```python
from build123d import *

# Parameters (mm, degrees)
SKETCH1_W           = 274
SKETCH1_H           = 180
SKETCH1_R           = 1.4
SKETCH1_R_2         = 16
SKETCH1_R_3         = 5
SKETCH1_R_4         = 3.15
SKETCH1_R_5         = 1.65
BOSS_EXTRUDE1_DEPTH = 6


with BuildPart() as part:
    # Sketch1 → Boss-Extrude1 (new body)
    with BuildSketch(Plane(origin=(0, 0, 0), x_dir=(1, 0, 0), z_dir=(0, 1, 0))):
        Rectangle(SKETCH1_W, SKETCH1_H)
        with Locations(Location((-75, -3, 0), (0, 0, 270))):
            Circle(SKETCH1_R, mode=Mode.SUBTRACT)
        with Locations(Location((-87, -15, 0), (0, 0, 270))):
            Circle(SKETCH1_R, mode=Mode.SUBTRACT)
        with Locations(Location((-75, -27, 0), (0, 0, 270))):
            Circle(SKETCH1_R, mode=Mode.SUBTRACT)
        with Locations(Location((-37, -15, 0), (0, 0, 270))):
            Circle(SKETCH1_R_2, mode=Mode.SUBTRACT)
        with Locations(Location((-58, -21, 0), (0, 0, 270))):
            Circle(SKETCH1_R_3, mode=Mode.SUBTRACT)
        with Locations(Location((-99.5, 5, 0), (0, 0, 270))):
            Circle(SKETCH1_R_4, mode=Mode.SUBTRACT)
        with Locations(Location((24.097224397, 76.923560319, 0), (0, 0, 270))):
            Circle(SKETCH1_R_4, mode=Mode.SUBTRACT)
        with Locations(Location((5.5, -7.5, 0), (0, 0, 270))):
            Circle(SKETCH1_R_4, mode=Mode.SUBTRACT)
        with Locations(Location((44.241196746, -7.5, 0), (0, 0, 270))):
            Circle(SKETCH1_R_4, mode=Mode.SUBTRACT)
        with Locations(Location((57.102540378, 42.5, 0), (0, 0, 270))):
            Circle(SKETCH1_R_4, mode=Mode.SUBTRACT)
        with Locations(Location((101.504885591, 27.217533736, 0), (0, 0, 270))):
            Circle(SKETCH1_R_4, mode=Mode.SUBTRACT)
        with Locations(Location((112.15381179, 65.773990664, 0), (0, 0, 270))):
            Circle(SKETCH1_R_4, mode=Mode.SUBTRACT)
        with Locations(Location((90.5, -85, 0), (0, 0, 270))):
            Circle(SKETCH1_R_4, mode=Mode.SUBTRACT)
        with Locations(Location((-4.5, -85, 0), (0, 0, 270))):
            Circle(SKETCH1_R_4, mode=Mode.SUBTRACT)
        with Locations(Location((-99.5, -85, 0), (0, 0, 270))):
            Circle(SKETCH1_R_4, mode=Mode.SUBTRACT)
        with Locations(Location((-122, 60.49863196, 0), (0, 0, 270))):
            Circle(SKETCH1_R_5, mode=Mode.SUBTRACT)
        with Locations(Location((-122, 34.50136804, 0), (0, 0, 270))):
            Circle(SKETCH1_R_5, mode=Mode.SUBTRACT)
        with Locations(Location((-117, -60, 0), (0, 0, 270))):
            Circle(SKETCH1_R_4, mode=Mode.SUBTRACT)
        with Locations(Location((-47, -60, 0), (0, 0, 270))):
            Circle(SKETCH1_R_4, mode=Mode.SUBTRACT)
        with Locations(Location((7, -61.482471058, 0), (0, 0, 270))):
            Circle(SKETCH1_R_4, mode=Mode.SUBTRACT)
        with Locations(Location((117, -61.482471058, 0), (0, 0, 270))):
            Circle(SKETCH1_R_4, mode=Mode.SUBTRACT)
        with Locations(Location((132, 50, 0), (0, 0, 270))):
            Circle(SKETCH1_R_5, mode=Mode.SUBTRACT)
        with Locations(Location((132, 30, 0), (0, 0, 270))):
            Circle(SKETCH1_R_5, mode=Mode.SUBTRACT)
        with Locations(Location((132, 10, 0), (0, 0, 270))):
            Circle(SKETCH1_R_5, mode=Mode.SUBTRACT)
        with Locations(Location((132, -10, 0), (0, 0, 270))):
            Circle(SKETCH1_R_5, mode=Mode.SUBTRACT)
        with Locations(Location((132, -30, 0), (0, 0, 270))):
            Circle(SKETCH1_R_5, mode=Mode.SUBTRACT)
        with Locations(Location((132, -50, 0), (0, 0, 270))):
            Circle(SKETCH1_R_5, mode=Mode.SUBTRACT)
        with Locations(Location((132, -70, 0), (0, 0, 270))):
            Circle(SKETCH1_R_5, mode=Mode.SUBTRACT)
        with Locations(Location((112, 50, 0), (0, 0, 270))):
            Circle(SKETCH1_R_5, mode=Mode.SUBTRACT)
        with Locations(Location((112, -10, 0), (0, 0, 270))):
            Circle(SKETCH1_R_5, mode=Mode.SUBTRACT)
        with Locations(Location((112, -30, 0), (0, 0, 270))):
            Circle(SKETCH1_R_5, mode=Mode.SUBTRACT)
        with Locations(Location((112, -50, 0), (0, 0, 270))):
            Circle(SKETCH1_R_5, mode=Mode.SUBTRACT)
        with Locations(Location((112, -70, 0), (0, 0, 270))):
            Circle(SKETCH1_R_5, mode=Mode.SUBTRACT)
        with Locations(Location((92, 50, 0), (0, 0, 270))):
            Circle(SKETCH1_R_5, mode=Mode.SUBTRACT)
        with Locations(Location((92, 30, 0), (0, 0, 270))):
            Circle(SKETCH1_R_5, mode=Mode.SUBTRACT)
        with Locations(Location((92, 10, 0), (0, 0, 270))):
            Circle(SKETCH1_R_5, mode=Mode.SUBTRACT)
        with Locations(Location((92, -30, 0), (0, 0, 270))):
            Circle(SKETCH1_R_5, mode=Mode.SUBTRACT)
        with Locations(Location((92, -50, 0), (0, 0, 270))):
            Circle(SKETCH1_R_5, mode=Mode.SUBTRACT)
        with Locations(Location((72, 50, 0), (0, 0, 270))):
            Circle(SKETCH1_R_5, mode=Mode.SUBTRACT)
        with Locations(Location((72, 30, 0), (0, 0, 270))):
            Circle(SKETCH1_R_5, mode=Mode.SUBTRACT)
        with Locations(Location((72, 10, 0), (0, 0, 270))):
            Circle(SKETCH1_R_5, mode=Mode.SUBTRACT)
        with Locations(Location((72, -30, 0), (0, 0, 270))):
            Circle(SKETCH1_R_5, mode=Mode.SUBTRACT)
        with Locations(Location((72, -50, 0), (0, 0, 270))):
            Circle(SKETCH1_R_5, mode=Mode.SUBTRACT)
        with Locations(Location((52, -30, 0), (0, 0, 270))):
            Circle(SKETCH1_R_5, mode=Mode.SUBTRACT)
        with Locations(Location((52, -50, 0), (0, 0, 270))):
            Circle(SKETCH1_R_5, mode=Mode.SUBTRACT)
        with Locations(Location((32, 30, 0), (0, 0, 270))):
            Circle(SKETCH1_R_5, mode=Mode.SUBTRACT)
        with Locations(Location((32, 10, 0), (0, 0, 270))):
            Circle(SKETCH1_R_5, mode=Mode.SUBTRACT)
        with Locations(Location((32, -10, 0), (0, 0, 270))):
            Circle(SKETCH1_R_5, mode=Mode.SUBTRACT)
        with Locations(Location((32, -30, 0), (0, 0, 270))):
            Circle(SKETCH1_R_5, mode=Mode.SUBTRACT)
        with Locations(Location((32, -50, 0), (0, 0, 270))):
            Circle(SKETCH1_R_5, mode=Mode.SUBTRACT)
        with Locations(Location((12, 50, 0), (0, 0, 270))):
            Circle(SKETCH1_R_5, mode=Mode.SUBTRACT)
        with Locations(Location((12, 30, 0), (0, 0, 270))):
            Circle(SKETCH1_R_5, mode=Mode.SUBTRACT)
        with Locations(Location((12, 10, 0), (0, 0, 270))):
            Circle(SKETCH1_R_5, mode=Mode.SUBTRACT)
        with Locations(Location((12, -30, 0), (0, 0, 270))):
            Circle(SKETCH1_R_5, mode=Mode.SUBTRACT)
        with Locations(Location((12, -50, 0), (0, 0, 270))):
            Circle(SKETCH1_R_5, mode=Mode.SUBTRACT)
        with Locations(Location((-8, 50, 0), (0, 0, 270))):
            Circle(SKETCH1_R_5, mode=Mode.SUBTRACT)
        with Locations(Location((-8, 30, 0), (0, 0, 270))):
            Circle(SKETCH1_R_5, mode=Mode.SUBTRACT)
        with Locations(Location((-8, 10, 0), (0, 0, 270))):
            Circle(SKETCH1_R_5, mode=Mode.SUBTRACT)
        with Locations(Location((-8, -30, 0), (0, 0, 270))):
            Circle(SKETCH1_R_5, mode=Mode.SUBTRACT)
        with Locations(Location((-8, -50, 0), (0, 0, 270))):
            Circle(SKETCH1_R_5, mode=Mode.SUBTRACT)
        with Locations(Location((-28, 50, 0), (0, 0, 270))):
            Circle(SKETCH1_R_5, mode=Mode.SUBTRACT)
        with Locations(Location((-28, 30, 0), (0, 0, 270))):
            Circle(SKETCH1_R_5, mode=Mode.SUBTRACT)
        with Locations(Location((-28, -50, 0), (0, 0, 270))):
            Circle(SKETCH1_R_5, mode=Mode.SUBTRACT)
        with Locations(Location((-48, 50, 0), (0, 0, 270))):
            Circle(SKETCH1_R_5, mode=Mode.SUBTRACT)
        with Locations(Location((-48, 30, 0), (0, 0, 270))):
            Circle(SKETCH1_R_5, mode=Mode.SUBTRACT)
        with Locations(Location((-48, -50, 0), (0, 0, 270))):
            Circle(SKETCH1_R_5, mode=Mode.SUBTRACT)
        with Locations(Location((-68, 50, 0), (0, 0, 270))):
            Circle(SKETCH1_R_5, mode=Mode.SUBTRACT)
        with Locations(Location((-68, 30, 0), (0, 0, 270))):
            Circle(SKETCH1_R_5, mode=Mode.SUBTRACT)
        with Locations(Location((-68, -50, 0), (0, 0, 270))):
            Circle(SKETCH1_R_5, mode=Mode.SUBTRACT)
        with Locations(Location((-88, 50, 0), (0, 0, 270))):
            Circle(SKETCH1_R_5, mode=Mode.SUBTRACT)
        with Locations(Location((-88, 30, 0), (0, 0, 270))):
            Circle(SKETCH1_R_5, mode=Mode.SUBTRACT)
        with Locations(Location((-88, -50, 0), (0, 0, 270))):
            Circle(SKETCH1_R_5, mode=Mode.SUBTRACT)
        with Locations(Location((-108, 50, 0), (0, 0, 270))):
            Circle(SKETCH1_R_5, mode=Mode.SUBTRACT)
        with Locations(Location((-108, 30, 0), (0, 0, 270))):
            Circle(SKETCH1_R_5, mode=Mode.SUBTRACT)
        with Locations(Location((-108, -10, 0), (0, 0, 270))):
            Circle(SKETCH1_R_5, mode=Mode.SUBTRACT)
        with Locations(Location((-108, -30, 0), (0, 0, 270))):
            Circle(SKETCH1_R_5, mode=Mode.SUBTRACT)
        with Locations(Location((-108, -50, 0), (0, 0, 270))):
            Circle(SKETCH1_R_5, mode=Mode.SUBTRACT)
        with Locations(Location((-128, -10, 0), (0, 0, 270))):
            Circle(SKETCH1_R_5, mode=Mode.SUBTRACT)
        with Locations(Location((-128, -30, 0), (0, 0, 270))):
            Circle(SKETCH1_R_5, mode=Mode.SUBTRACT)
        with Locations(Location((-128, -50, 0), (0, 0, 270))):
            Circle(SKETCH1_R_5, mode=Mode.SUBTRACT)
    extrude(amount=BOSS_EXTRUDE1_DEPTH)


solid = part.part
```
Design review of the part built by this model. Coordinates are the model's own, in mm. Coordinates: 2 decimals unless noted, no trailing zeros. Write each loop counter-clockwise with the first axis right and the second up, starting at its lowest first coordinate (ties: lowest second). Pieces come first, ordered by that corner, then holes.
1) Mouldability with a two-part tool opening along Z and no side actions: class faces 1 (the cylindrical face through (7.138, 2.958, 58.336)), 2 (the flat face through (137, 3, 1)) as +Z half, -Z half, draft (parallel to the pull), parting line (faces both ways), or undercut.
2) Add section B-B (z = -42.5). Write out the cut boundary in (x, y).
3) To check wall thickness, follow L1, parallel to X at y = 4.8, z = 70; L2, parallel to Z at x = -74.5, y = 5.7; L3, parallel to Z at x = 33, y = 5.55. State the ranges of each line that lie inside material, in increasing order.
4) Add section C-C (y = 4.4). State how many separate pieces and enclosed holes the cut face has, plus the area to 3 significant figures.
5) Add section A-A (x = -117). Write out the cut boundary in (y, z).
Check result:
1. face 1: undercut
1. face 2: draft
2. outline: (-137, 0) - (53.95, 0) - (53.95, 6) - (-137, 6) - close; (60.25, 0) - (137, 0) - (137, 6) - (60.25, 6) - close
3. L1: x = -137 to 110.35, 113.65 to 130.35, 133.65 to 137
3. L2: z = -90 to 1.69, 4.31 to 25.69, 28.31 to 90
3. L3: z = -90 to -31.31, -28.69 to -11.31, -8.69 to 8.69, 11.31 to 28.69, 31.31 to 48.69, 51.31 to 90
4. separate pieces: 1
4. enclosed holes: 80
4. area: 47,500 mm2
5. outline: (0, -90) - (6, -90) - (6, 56.85) - (0, 56.85) - close; (0, 63.15) - (6, 63.15) - (6, 90) - (0, 90) - close
